from build123d import *

# Parameters (mm, degrees)
BOSS_EXTRUDE1_DEPTH = 3
SKETCH2_W           = 109.999996871
SKETCH2_H           = 44.999998436
CUT_EXTRUDE1_DEPTH  = 10


with BuildPart() as part:
    # Sketch1 → Boss-Extrude1 (new body)
    with BuildSketch(Plane.XY):
        Polygon((158.754970941, -72.897106565), (180.070576123, -94.00741153), (180.070576123, -95.284756679), (178.131724855, -97.223607947), (175.233947376, -96.447150811), (148.786793436, -69.999996871), (21.213203436, -69.999996871), (-5.233950505, -96.447150811), (-8.131727984, -97.223607947), (-10.070579252, -95.284756679), (-10.070579252, -94.00741153), (11.24502593, -72.897106565), (-2.828675487, -58.686536734), (-24.144280669, -79.796841699), (-25.558494231, -79.796841699), (-27.223611076, -78.131724855), (-26.44715394, -75.233947376), (0, -48.786793435), (0, 78.786796565), (-26.44715394, 105.233950505), (-27.223611076, 108.131727984), (-25.558494231, 109.796844828), (-24.144280669, 109.796844828), (-2.828675487, 88.686539863), (11.24502593, 102.897109694), (-10.070579252, 124.007414659), (-10.070579252, 125.284759808), (-8.131727984, 127.223611076), (-5.233950505, 126.447153941), (21.213203436, 100), (148.786793436, 100), (175.233947376, 126.447153941), (178.131724855, 127.223611076), (180.070576123, 125.284759808), (180.070576123, 124.007414659), (158.754970941, 102.897109694), (172.828672358, 88.686539863), (194.14427754, 109.796844828), (195.558491102, 109.796844828), (197.223607947, 108.131727984), (196.447150812, 105.233950505), (169.999996871, 78.786796565), (169.999996871, -48.786793435), (196.447150812, -75.233947376), (197.223607947, -78.131724855), (195.558491102, -79.796841699), (194.14427754, -79.796841699), (172.828672358, -58.686536734), align=None)
    extrude(amount=BOSS_EXTRUDE1_DEPTH)

    # Sketch2 → Cut-Extrude1 (cut)
    with BuildSketch(Plane.XY.offset(3)):
        Polygon((30, 70), (40, 80), (54.999998436, 80), (54.999998436, 37.500001565), (52.499998436, 35.000001565), (30, 35.000001565), align=None)
        Polygon((139.999996871, 35.000001565), (117.499998436, 35.000001565), (114.999998436, 37.500001565), (114.999998436, 80), (129.999996871, 80), (139.999996871, 70), align=None)
        with Locations((84.999998436, -22.499997653)):
            Rectangle(SKETCH2_W, SKETCH2_H)
    extrude(amount=-CUT_EXTRUDE1_DEPTH, mode=Mode.SUBTRACT)


solid = part.part
For this review, take the finished solid that the model builds, in its own axes (mm). A direction names the side the tool comes from. Round coordinates to 2 decimals unless told otherwise and drop trailing zeros. Order: outer loops, then holes, each group sorted by start corner. A loop starts at its lowest first (then second) coordinate and runs counter-clockwise, first axis right, second up. Notation, with made-up numbers: (71, -6.5) -> (112, -6.5) arc R18 cw to (112, 9.5) -> close; hole circle Ø10 at (21.25, 18.5). An arc over 180 degrees is marked (long way). Write item = value, one per line. Start each with the question number.
1) The part is to be moulded in two halves that separate along Y. For faces 1 (the face through (7.804, 113.409, 1.479)), 2 (the face through (169.56, 113.6, 1.48)), 3 (the face through (183.636, -69.389, 1.479)), 4 (the face through (87, 17, 0)), say which applies: +Y half, -Y half, draft (parallel to the pull), parting line (faces both ways), or undercut.
2) Take a section at C-C on y = 60. State the section outline as (x, z) points, plus the area to 3 significant figures.
3) Insertion check: pin 1 (0.6 mm diameter, centred on y = -95, z = 1.5, fed in from -X); pin 2 (1.5 mm diameter, centred on x = 128, z = 2, fed in from +Y); pin 3 (1.1 mm diameter, centred on x = -25, z = 1, fed in from -Y). Each pin has a flat end and moves straight along its axis. Give the tip position at first contact, or say it passes through.
4) Tool access review of faces 5 (the face through (165.693, 95.891, 1.479)), 6 (the face through (183.038, -61.825, 1.479)), 7 (the face through (-13.409, -62.196, 1.479)): name each direction out of +Z, -Z, +X, -X, +Y, -Y from which nothing blocks a thin tool from reaching the whole face with its end or side.
5) Take a section at B-B on y = -9. State the section outline as (x, z) points.
6) Take a section at D-D on x = 165. State the section outline as (y, z) points, plus the area to 3 significant figures.
7) Take a section at A-A on x = 98.5. State the section outline as (y, z) points.
8) To check wall thickness, follow line 1 (X direction, y = 43, z = 2.25); line 2 (Y direction, x = 125.5, z = 1.4); line 3 (Y direction, x = 69, z = 2.6). State the ranges of each line that lie inside material, in increasing order. Write a range as from..to.
Verdict:
q1.face_1 = +Y half
q1.face_2 = undercut
q1.face_3 = undercut
q1.face_4 = draft
q2.outline = (0, 0) -> (30, 0) -> (30, 3) -> (0, 3) -> close; (55, 0) -> (115, 0) -> (115, 3) -> (55, 3) -> close; (140, 0) -> (170, 0) -> (170, 3) -> (140, 3) -> close
q2.area = 360 mm2
q3.pin_1 = -10.07
q3.pin_2 = 100
q3.pin_3 = -79.8
q4.face_5 = +Z, -Z
q4.face_6 = +Z, -Z, +X
q4.face_7 = +Z, -Z, -X
q5.outline = (0, 0) -> (30, 0) -> (30, 3) -> (0, 3) -> close; (140, 0) -> (170, 0) -> (170, 3) -> (140, 3) -> close
q6.outline = (-86.21, 0) -> (-79.08, 0) -> (-79.08, 3) -> (-86.21, 3) -> close; (-66.59, 0) -> (96.59, 0) -> (96.59, 3) -> (-66.59, 3) -> close; (109.08, 0) -> (116.21, 0) -> (116.21, 3) -> (109.08, 3) -> close
q6.area = 532 mm2
q7.outline = (-70, 0) -> (-45, 0) -> (-45, 3) -> (-70, 3) -> close; (0, 0) -> (100, 0) -> (100, 3) -> (0, 3) -> close
q8.line_1 = 0..30, 55..115, 140..170
q8.line_2 = -70..-45, 0..35, 80..100
q8.line_3 = -70..-45, 0..100
